Could you check a few things on this model? Use its own coordinates, in mm. Give positions to 0.01 mm unless a question says otherwise; leave off trailing zeros. Order: outer loops, then holes, each group sorted by start corner. A loop starts at its lowest first (then second) coordinate and runs counter-clockwise, first axis right, second up. Notation, with made-up numbers: (76.5, 39.5) - (107.5, 39.5) arc R11 ccw to (107.5, 58.5) - close; hole circle Ø2 at (3.5, 81). An arc over 180 degrees is marked (long way). Put each result on its own line as item: value.
from build123d import *

# Parameters (mm, degrees)
EXTRUDE1_DEPTH     = 1.56
SKETCH2_R          = 1.3462
CUT_EXTRUDE2_DEPTH = 2.56
SKETCH3_R          = 0.396875
EXTRUDE2_DEPTH     = 1.56
FILLET1_R          = 0.5


with BuildPart() as part:
    # Sketch1 → Extrude1 (new body)
    with BuildSketch(Plane.XY):
        Polygon((-7.655500535, 35), (7.655500535, 35), (11.535673534, 94.2), (-11.535673534, 94.2), align=None)
    extrude(amount=EXTRUDE1_DEPTH)

    # Sketch2 → Cut-Extrude2 (cut, through all)
    with BuildSketch(Plane(origin=(2.513247729, -24.95744912, 1.56), x_dir=(1, 0, 0), z_dir=(0, 0, 1))):
        with Locations((-2.513247729, 66.45744912)):
            Circle(SKETCH2_R)
    extrude(amount=-CUT_EXTRUDE2_DEPTH, mode=Mode.SUBTRACT)

    # Sketch3 → Extrude2 (add)
    with BuildSketch(Plane.XY.offset(1.56)):
        with BuildLine():
            Line((11.535673534, 94.2), (7.646607283, 94.2))
            Line((7.646607283, 94.2), (7.646607283, 95.22402761))
            ThreePointArc((7.646607283, 95.22402761), (9.687231677, 97.19894204), (11.594321354, 95.094792832))
            Line((11.594321354, 95.094792832), (11.535673534, 94.2))
        make_face()
        with Locations((9.622579673, 95.22402761)):
            Circle(SKETCH3_R, mode=Mode.SUBTRACT)
    extrude(amount=-EXTRUDE2_DEPTH)

    # Fillet1
    fillet1_edges = [part.edges().sort_by_distance(p)[0] for p in [
        (7.646607283, 94.2, 0.78),
    ]]
    fillet(fillet1_edges, radius=FILLET1_R)


solid = part.part
1) We'd pull the mould along Y, two halves only. Please class faces 1 (the flat face through (0, 67, 0)), 2 (the flat face through (-2, 94.2, 1)), 3 (the cylindrical face through (-0.175, 42.835, 0.791)), 4 (the flat face through (0, 35, 1)): pulls with the +Y half, pulls with the -Y half, needs draft (parallel to the pull), parting line crosses it, or undercut.
Filled in:
face 1: needs draft
face 2: pulls with the +Y half
face 3: undercut
face 4: pulls with the -Y half
2) If I drill on line 1 (Y direction, x = 0, z = 0.4); line 2 (Y direction, x = -3.25, z = 0.7); line 3 (Y direction, x = 0.5, z = 1.45), over which ranges is the centre line in solid material (lowest first)? Write a range as [from, to].
Filled in:
line 1: y = [35, 40.15], [42.85, 94.2]
line 2: y = [35, 94.2]
line 3: y = [35, 40.25], [42.75, 94.2]
3) Suppose I cut it at C-C, the plane y = 41.5. List the corners of the cut face in (x, z) for me, and give its area (3 significant figures).
Filled in:
outline: (-8.08, 0) - (-1.35, 0) - (-1.35, 1.56) - (-8.08, 1.56) - close; (1.35, 0) - (8.08, 0) - (8.08, 1.56) - (1.35, 1.56) - close
area: 21.0 mm^2
4) Suppose I cut it at D-D, the plane x = -5. List the corners of the cut face in (y, z) for me, and give its area (3 significant figures).
Filled in:
outline: (35, 0) - (94.2, 0) - (94.2, 1.56) - (35, 1.56) - close
area: 92.4 mm^2
5) Suppose I cut it at A-A, the plane z = 1.1. List the corners of the cut face in (x, y) for me, and give its area (3 significant figures).
Filled in:
outline: (-11.54, 94.2) - (-7.66, 35) - (7.66, 35) - (11.59, 95.09) arc R1.98 ccw (long way) to (7.65, 95.22) - (7.65, 94.7) arc R0.5 cw to (7.15, 94.2) - close; hole circle Ø2.69 at (0, 41.5); hole circle Ø0.79 at (9.62, 95.22)
area: 1,140 mm^2
6) Suppose I cut it at B-B, the plane x = 0. List the corners of the cut face in (y, z) for me.
Filled in:
outline: (35, 0) - (40.15, 0) - (40.15, 1.56) - (35, 1.56) - close; (42.85, 0) - (94.2, 0) - (94.2, 1.56) - (42.85, 1.56) - close
